```python
from build123d import *

# Parameters (mm, degrees)
ESBO_O1_W                = 280
ESBO_O1_H                = 110
RESSALTO_EXTRUS_O1_DEPTH = 3
CORTE_EXTRUS_O1_DEPTH    = 280
ESBO_O4_R                = 4
RESSALTO_EXTRUS_O2_DEPTH = 60


with BuildPart() as part:
    # Esboço1 → Ressalto-extrusão1 (new body)
    with BuildSketch(Plane.XY):
        Rectangle(ESBO_O1_W, ESBO_O1_H)
    extrude(amount=RESSALTO_EXTRUS_O1_DEPTH)

    # Esboço3 → Corte-extrusão1 (cut)
    with BuildSketch(Plane.ZY.offset(140)):
        Polygon((0, -55), (3.02401214, -30.57), (3, -55), align=None)
    extrude(amount=-CORTE_EXTRUS_O1_DEPTH, mode=Mode.SUBTRACT)

    # Esboço4 → Ressalto-extrusão2 (add)
    with BuildSketch(Plane.XY.offset(3)):
        with Locations(Location((134.2, 49.8, 0), (0, 0, 180))):
            Circle(ESBO_O4_R)
        with Locations(Location((67.1, 49.8, 0), (0, 0, 180))):
            Circle(ESBO_O4_R)
        with Locations(Location((0, 49.8, 0), (0, 0, 180))):
            Circle(ESBO_O4_R)
        with Locations(Location((-67.1, 49.8, 0), (0, 0, 180))):
            Circle(ESBO_O4_R)
        with Locations(Location((-134.2, 49.8, 0), (0, 0, 180))):
            Circle(ESBO_O4_R)
        with Locations(Location((-134.2, -25.563986188, 0), (0, 0, 180))):
            Circle(ESBO_O4_R)
        with Locations(Location((-67.1, -25.563986188, 0), (0, 0, 180))):
            Circle(ESBO_O4_R)
        with Locations(Location((0, -25.563986188, 0), (0, 0, 180))):
            Circle(ESBO_O4_R)
        with Locations(Location((67.1, -25.563986188, 0), (0, 0, 180))):
            Circle(ESBO_O4_R)
        with Locations(Location((134.2, -25.563986188, 0), (0, 0, 180))):
            Circle(ESBO_O4_R)
    extrude(amount=RESSALTO_EXTRUS_O2_DEPTH)


solid = part.part
```
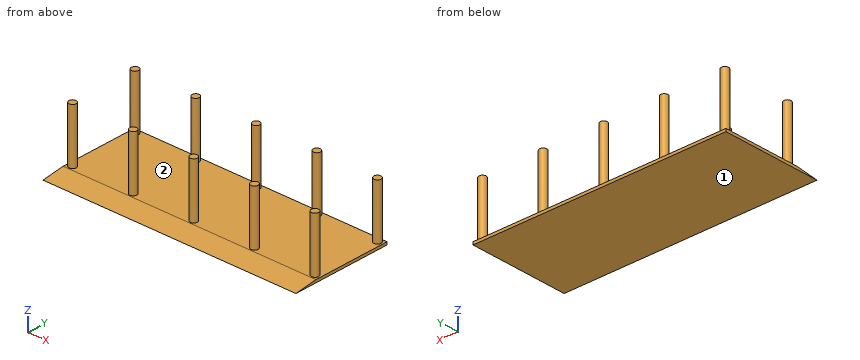
The listing builds one solid part. Answer for the finished solid, in the listing's coordinates (mm). Face numbers are marked on the shaded views. Coordinates: 2 decimals unless noted, no trailing zeros. Loops run counter-clockwise (first coordinate to the right, second up) from the corner with the lowest first, then second, coordinate; pieces in that order, holes last. Notation, with made-up numbers: (47, 54.5) - (98, 54.5) arc R15 cw to (98, 77.5) - close; hole circle Ø1 at (75, 31). An arc over 180 degrees is marked (long way). Write item = value, one per line.
1) Determine the mould class of the marked faces 1 and 2 for opening direction X: pulls with the +X half, pulls with the -X half, needs draft (parallel to the pull), parting line crosses it, or undercut.
Responses:
face_1 = needs draft
face_2 = undercut
2) Section A-A (z = 21) is taken. Count the separate pieces of the cut face and the enclosed holes in it, plus the area to 3 significant figures.
Responses:
separate_pieces = 10
enclosed_holes = 0
area = 503 mm^2
3) Section D-D (x = -93.5) is taken. Determine the outline of the cut face in (y, z), plus the area to 3 significant figures.
Responses:
outline = (-55, 0) - (55, 0) - (55, 3) - (-30.76, 3) - close
area = 294 mm^2
4) Section B-B (x = -134.2) is taken. Determine the outline of the cut face in (y, z), plus the area to 3 significant figures.
Responses:
outline = (-55, 0) - (55, 0) - (55, 3) - (53.8, 3) - (53.8, 63) - (45.8, 63) - (45.8, 3) - (-21.56, 3) - (-21.56, 63) - (-29.56, 63) - (-29.56, 3) - (-30.76, 3) - close
area = 1,250 mm^2
5) Each of these flat-tipped pins is pushed along its axis until it touches: P1, Ø6, axis at x = 6.5, y = -14.5, coming from the +Z side; P2, Ø12, axis at x = 61.5, y = -26, coming from the +Z side; P3, Ø5, axis at x = 2, z = 47.5, coming from the -Y side. Where does it stop, or does it pass through?
Responses:
P1 = 3
P2 = 63
P3 = -29.56
6) Section C-C (y = -47.5) is taken. Determine the outline of the cut face in (x, z), plus the area to 3 significant figures.
Responses:
outline = (-140, 0) - (140, 0) - (140, 0.93) - (-140, 0.93) - close
area = 260 mm^2
7) Find the intervals of material crossed by line 1 along X through (y, z) = (50, 49.5) (3 decimals); line 2 along Z through (x, y) = (118.5, 0.5); line 3 along Y through (x, z) = (64, 34.5), in increasing order.
Responses:
line_1 = -138.195 to -130.205, -71.095 to -63.105, -3.995 to 3.995, 63.105 to 71.095, 130.205 to 138.195
line_2 = 0 to 3
line_3 = -28.09 to -23.04, 47.27 to 52.33
